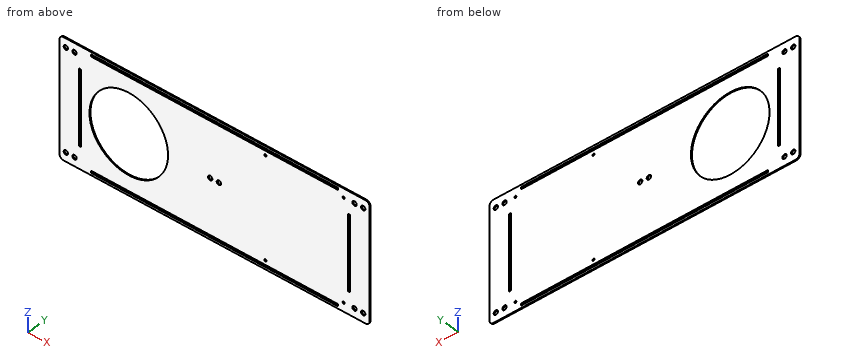
```python
from build123d import *

# Parameters (mm, degrees)
SKETCH1_W           = 454.025
SKETCH1_H           = 171.45
BOSS_EXTRUDE1_DEPTH = 1.5875
FILLET1_R           = 6.35
SKETCH3_W           = 361.95
SKETCH3_H           = 3.175
SKETCH3_W_2         = 3.175
SKETCH3_H_2         = 107.95
CUT_EXTRUDE1_DEPTH  = 486.320845711
SKETCH4_R           = 3.175
CUT_EXTRUDE2_DEPTH  = 486.320845711
SKETCH6_R           = 1.5875
CUT_EXTRUDE3_DEPTH  = 486.320845711
SKETCH7_R           = 57.5
CUT_EXTRUDE4_DEPTH  = 486.320845711


with BuildPart() as part:
    # Sketch1 → Boss-Extrude1 (new body)
    with BuildSketch(Plane(origin=(0, 0, 0), x_dir=(1, 0, 0), z_dir=(0, 1, 0))):
        with Locations((227.0125, 85.725)):
            Rectangle(SKETCH1_W, SKETCH1_H)
    extrude(amount=BOSS_EXTRUDE1_DEPTH)

    # Fillet1
    fillet1_edges = [part.edges().sort_by_distance(p)[0] for p in [
        (0, 0.79375, -171.45),
        (454.025, 0.79375, -171.45),
        (454.025, 0.79375, 0),
        (0, 0.79375, 0),
    ]]
    fillet(fillet1_edges, radius=FILLET1_R)

    # Sketch3 → Cut-Extrude1 (cut, through all)
    with BuildSketch(Plane(origin=(0, 1.5875, 0), x_dir=(1, 0, 0), z_dir=(0, 1, 0))):
        with Locations((227.0125, 166.6875)):
            Rectangle(SKETCH3_W, SKETCH3_H)
        with Locations((30.1625, 85.725)):
            Rectangle(SKETCH3_W_2, SKETCH3_H_2)
        with Locations((227.0125, 4.7625)):
            Rectangle(SKETCH3_W, SKETCH3_H)
        with Locations((423.8625, 85.725)):
            Rectangle(SKETCH3_W_2, SKETCH3_H_2)
    extrude(amount=-CUT_EXTRUDE1_DEPTH, mode=Mode.SUBTRACT)

    # Sketch4 → Cut-Extrude2 (cut, through all)
    with BuildSketch(Plane(origin=(0, 1.5875, 0), x_dir=(1, 0, 0), z_dir=(0, 1, 0))):
        with Locations(Location((9.525, 158.75, 0), (0, 0, 270))):
            Circle(SKETCH4_R)
        with Locations(Location((22.225, 158.75, 0), (0, 0, 270))):
            Circle(SKETCH4_R)
        with Locations(Location((431.8, 158.75, 0), (0, 0, 270))):
            Circle(SKETCH4_R)
        with Locations(Location((444.5, 158.75, 0), (0, 0, 270))):
            Circle(SKETCH4_R)
        with Locations(Location((431.8, 12.7, 0), (0, 0, 270))):
            Circle(SKETCH4_R)
        with Locations(Location((444.5, 12.7, 0), (0, 0, 270))):
            Circle(SKETCH4_R)
        with Locations(Location((9.525, 12.7, 0), (0, 0, 270))):
            Circle(SKETCH4_R)
        with Locations(Location((22.225, 12.7, 0), (0, 0, 270))):
            Circle(SKETCH4_R)
        with Locations(Location((220.6625, 85.725, 0), (0, 0, 270))):
            Circle(SKETCH4_R)
        with Locations(Location((233.3625, 85.725, 0), (0, 0, 270))):
            Circle(SKETCH4_R)
    extrude(amount=-CUT_EXTRUDE2_DEPTH, mode=Mode.SUBTRACT)

    # Sketch6 → Cut-Extrude3 (cut, through all)
    with BuildSketch(Plane(origin=(0, 1.5875, 0), x_dir=(1, 0, 0), z_dir=(0, 1, 0))):
        with Locations(Location((301.625, 158.75, 0), (0, 0, 270))):
            Circle(SKETCH6_R)
        with Locations(Location((415.925, 158.75, 0), (0, 0, 270))):
            Circle(SKETCH6_R)
        with Locations(Location((415.925, 12.7, 0), (0, 0, 270))):
            Circle(SKETCH6_R)
        with Locations(Location((301.625, 12.7, 0), (0, 0, 270))):
            Circle(SKETCH6_R)
    extrude(amount=-CUT_EXTRUDE3_DEPTH, mode=Mode.SUBTRACT)

    # Sketch7 → Cut-Extrude4 (cut, through all)
    with BuildSketch(Plane(origin=(0, 1.5875, 0), x_dir=(1, 0, 0), z_dir=(0, 1, 0))):
        with Locations(Location((101.6, 85.725, 0), (0, 0, 270))):
            Circle(SKETCH7_R)
    extrude(amount=-CUT_EXTRUDE4_DEPTH, mode=Mode.SUBTRACT)


solid = part.part
```
The listing builds one solid part. Answer for the finished solid, in the listing's coordinates (mm). Round coordinates to 2 decimals unless told otherwise and drop trailing zeros. Answer as a JSON object with one key per item and string values. Group by question number.
Q1. Straight lines are drawn through the part: line 1 along Z through (x, y) = (203, 1.4) (3 decimals); line 2 along X through (y, z) = (0.15, -85.5) (3 decimals); line 3 along Z through (x, y) = (444.5, 0.65) (3 decimals). For each, find the intervals that lie inside material, in ascending order.
Q2. Section A-A (x = 324) is taken. Count the separate pieces of the cut face and the enclosed holes in it, plus the area to 3 significant figures.
Q3. Each of these flat-tipped pins is pushed along its axis until it touches: pin 1 Ø1.9 at (x, z) = (415.925, -12.7) entering from +Y (3 decimals); pin 2 Ø0.8 at (y, z) = (0.5, -5) entering from -X. Where does it stop, or does it pass through?
Check values:
{
 "1": {"line 1": "-171.45 to -168.275, -165.1 to -6.35, -3.175 to 0", "line 2": "0 to 28.575, 31.75 to 44.1, 159.1 to 217.495, 223.83 to 230.195, 236.53 to 422.275, 425.45 to 454.025", "line 3": "-171.45 to -161.925, -155.575 to -15.875, -9.525 to 0"},
 "2": {"separate pieces": "3", "enclosed holes": "0", "area": "262 mm^2"},
 "3": {"pin 1": "through", "pin 2": "x = 0.07"}
}
